Can you work these out from the model? Positions are in its coordinate system, mm. A direction names the side the tool comes from. Give positions to 0.01 mm unless a question says otherwise; leave off trailing zeros. Write each loop counter-clockwise with the first axis right and the second up, starting at its lowest first coordinate (ties: lowest second). Pieces come first, ordered by that corner, then holes.
1. Suppose I cut it at C-C (z = 6). Please give me the cut outline in (x, y), and give its area (3 significant figures).
2. On a 3-axis mill with a long thin cutter (end or side, diameter ignored), from which of +Z, -Z, +X, -X, +Y, -Y can I reach the whole of each face in a straight line? I mean faces 1 (the flat face through (40, -20, 5)), 2 (the flat face through (0, 3, 5)), 3 (the cylindrical face through (27.86, 4.52, 12.46)), 4 (the conical face through (28.08, -5.4, 1.85)), 5 (the cylindrical face through (27.315, -6.261, 4.972)). Say none if no direction works.
3. Suppose I cut it at A-A (x = 18). Please give me the cut outline in (y, z), and give its area (3 significant figures).
4. Thinking about a two-plate mould opening in X: for faces 6 (the cylindrical face through (-27.39, -6.33, 4.97)), 7 (the cylindrical face through (42.47, 18.01, 5.11)), 8 (the flat face through (-1, -1, 0)), which applies, pulls with the +X half, pulls with the -X half, needs draft (parallel to the pull), parting line crosses it, or undercut?
5. I'm going to push flat-ended pins straight in: pin 1 (1.5 mm diameter, centred on x = -27.5, y = -6, fed in from +Z); pin 2 (4.5 mm diameter, centred on x = -7.5, z = 5.5, fed in from -Y); pin 3 (3 mm diameter, centred on y = -2.5, z = 5.5, fed in from -X). Where does each tip first touch, or does it pass through?
6. If I drill on probe 1 along X at (y, z) = (10, 11.5); probe 2 along X at (y, z) = (10, 6.5); probe 3 along Y at (x, z) = (35, 7.5), over which ranges is the centre line in solid material (lowest first)?
7. Suppose I cut it at B-B (z = 11.75). Please give me the cut outline in (x, y).
```python
from build123d import *

# Parameters (mm, degrees)
F0_R     = 4
F1_DEPTH = 10
F2_R     = 9
F2_R_2   = 4
F3_DEPTH = 5
F4_R     = 4
F5_DEPTH = 3
F6_R     = 3
F7_SIZE  = 3


with BuildPart() as f1:
    # F0 (on Top) → F1 (new body)
    with BuildSketch(Plane.XY):
        with BuildLine():
            Line((32.279847, 22), (0, 22))
            Line((0, 22), (-32.279847, 22))
            ThreePointArc((-32.279847, 22), (-42.355492, 18.112218), (-47.208215, 8.464184))
            Line((-47.208215, 8.464184), (-50, -20))
            Line((-50, -20), (-30, -20))
            Line((-30, -20), (-28.971324, -9.511939))
            ThreePointArc((-28.971324, -9.511939), (-27.35375, -6.295927), (-23.995202, -5))
            Line((-23.995202, -5), (0, -5))
            Line((0, -5), (23.995202, -5))
            ThreePointArc((23.995202, -5), (27.35375, -6.295927), (28.971324, -9.511939))
            Line((28.971324, -9.511939), (30, -20))
            Line((30, -20), (50, -20))
            Line((50, -20), (47.208215, 8.464184))
            ThreePointArc((47.208215, 8.464184), (42.355492, 18.112218), (32.279847, 22))
        make_face()
        with Locations((-35, 10)):
            Circle(F0_R, mode=Mode.SUBTRACT)
        with BuildLine():
            Line((21.702398, 3), (0, 3))
            Line((0, 3), (-21.702398, 3))
            ThreePointArc((-21.702398, 3), (-23.346752, 3.861536), (-23.574435, 5.7039))
            ThreePointArc((-23.574435, 5.7039), (-22.990279, 7.816744), (-22.793444, 10))
            ThreePointArc((-22.793444, 10), (-21.914765, 12.12132), (-19.793444, 13))
            Line((-19.793444, 13), (19.793444, 13))
            ThreePointArc((19.793444, 13), (21.914765, 12.12132), (22.793444, 10))
            ThreePointArc((22.793444, 10), (22.990279, 7.816744), (23.574435, 5.7039))
            ThreePointArc((23.574435, 5.7039), (23.346752, 3.861536), (21.702398, 3))
        make_face(mode=Mode.SUBTRACT)
        with Locations((35, 10)):
            Circle(F0_R, mode=Mode.SUBTRACT)
    extrude(amount=F1_DEPTH)

    # F2 (on face) → F3 (join)
    with BuildSketch(Plane.XY.offset(10)):
        with Locations((35, 10)):
            Circle(F2_R)
        with Locations((35, 10)):
            Circle(F2_R_2, mode=Mode.SUBTRACT)
        with Locations((-35, 10)):
            Circle(F2_R)
        with Locations((-35, 10)):
            Circle(F2_R_2, mode=Mode.SUBTRACT)
    extrude(amount=F3_DEPTH)

    # F4 (on face) → F5 (join)
    with BuildSketch(Plane(origin=(0, 0, 0), x_dir=(1, 0, 0), z_dir=(0, 0, -1))):
        with Locations((35, -10)):
            Circle(F4_R)
        with Locations((-35, -10)):
            Circle(F4_R)
    extrude(amount=-F5_DEPTH)

    # F6
    f6_edges = [f1.edges().sort_by_distance(p)[0] for p in [
        (0, -5, 10),
        (0, 22, 10),
        (0, 13, 10),
    ]]
    fillet(f6_edges, radius=F6_R)

    # F7
    f7_edges = [f1.edges().sort_by_distance(p)[0] for p in [
        (42.355492, 18.112218, 0),
        (0, 13, 0),
        (0, -5, 0),
    ]]
    chamfer(f7_edges, length=F7_SIZE)


solid = f1.part
```
Checks:
1. outline: (-50, -20) - (-30, -20) - (-28.97, -9.51) arc R5 cw to (-24, -5) - (24, -5) arc R5 cw to (28.97, -9.51) - (30, -20) - (50, -20) - (47.21, 8.46) arc R15 ccw to (32.28, 22) - (-32.28, 22) arc R15 ccw to (-47.21, 8.46) - close; hole circle Ø8 at (-35, 10); hole (-23.57, 5.7) arc R2 ccw to (-21.7, 3) - (21.7, 3) arc R2 ccw to (23.57, 5.7) arc R12.21 cw to (22.79, 10) arc R3 ccw to (19.79, 13) - (-19.79, 13) arc R3 ccw to (-22.79, 10) arc R12.21 cw to start; hole circle Ø8 at (35, 10)
1. area: 2,520 mm2
2. face 1: +Z, -Z, +X, -X, -Y
2. face 2: +Z, -Z
2. face 3: +Z
2. face 4: -Z, -Y
2. face 5: +Z, -Z, -Y
3. outline: (-5, 3) - (-2, 0) - (0, 0) - (3, 3) - (3, 7) arc R3 ccw to (0, 10) - (-2, 10) arc R3 ccw to (-5, 7) - close; (13, 3) - (16, 0) - (19, 0) - (22, 3) - (22, 7) arc R3 ccw to (19, 10) - (16, 10) arc R3 ccw to (13, 7) - close
3. area: 144 mm2
4. face 6: undercut
4. face 7: pulls with the +X half
4. face 8: needs draft
5. pin 1: stops at z = 9.3
5. pin 2: stops at y = -5
5. pin 3: stops at x = -48.43
6. probe 1: x = -44 to -39, -31 to -26, 26 to 31, 39 to 44
6. probe 2: x = -46.98 to -39, -31 to -22.79, 22.79 to 31, 39 to 46.98
6. probe 3: y = -20 to 6, 14 to 21.71
7. outline: circle Ø18 at (-35, 10); circle Ø18 at (35, 10); hole circle Ø8 at (-35, 10); hole circle Ø8 at (35, 10)
